Design review of the part built by this model. Coordinates are the model's own, in mm. A direction names the side the tool comes from. Coordinates: 2 decimals unless noted, no trailing zeros. Order: outer loops, then holes, each group sorted by start corner. A loop starts at its lowest first (then second) coordinate and runs counter-clockwise, first axis right, second up. Notation, with made-up numbers: M 88.5,71 L 113.5,71 A30 ccw 113.5,98 Z; hole C -17,52.25 d5. An arc over 180 degrees is marked long. Use CSV: the item, a comma, the result in double quotes.
Autodesk Fusion 360 part; units mm, degrees
sketch "Sketch1" plane through (0, 0, 0) normal (0, 1, 0) x (1, 0, 0)
  line L0 (0, 0) -> (6, 0)
  line L1 (6, 0) -> (6, -6)
  line L2 (6, -6) -> (0, -6)
  line L3 (0, -6) -> (0, 0)
  dimension "d1" = 6
  dimension "d2" = 6
extrude "Extrude1" add sketch "Sketch1" along normal blind 1.9
sketch "Sketch2" plane through (0, 1.9, 0) normal (0, 1, 0) x (-1, 0, 0)
  line L0 (0, 6) -> (-6, 6)
  line L1 (-6, 6) -> (-6, 0)
  line L2 (-6, 0) -> (0, 0)
  line L3 (0, 0) -> (0, 6)
  line L4 (-1.7485, 1.7053) -> (-4.3485, 1.7053)
  line L5 (-4.3485, 1.7053) -> (-4.3485, 4.3053)
  line L6 (-4.3485, 4.3053) -> (-1.7485, 4.3053)
  line L7 (-1.7485, 4.3053) -> (-1.7485, 1.7053)
  dimension "d5" = 2.6
  dimension "d6" = 2.6
extrude "Extrude2" add sketch "Sketch2" along normal blind 6.2 contours L4 L5 L6 L7
sketch "Sketch3" plane through (0, 0, 0) normal (0, -1, 0) x (1, 0, 0)
  line L0 (6, 6) -> (0, 6)
  line L1 (0, 6) -> (0, 0)
  line L2 (0, 0) -> (6, 0)
  line L3 (6, 0) -> (6, 6)
  line L4 (1.7485, 4.3053) -> (4.3485, 4.3053)
  line L5 (4.3485, 4.3053) -> (4.3485, 1.7053)
  line L6 (4.3485, 1.7053) -> (1.7485, 1.7053)
  line L7 (1.7485, 1.7053) -> (1.7485, 4.3053)
  point P0 (1.7485, 4.3053)
  point P1 (4.3485, 1.7053)
extrude "Extrude3" add sketch "Sketch3" along normal blind 1 contours L4 L5 L6 L7
(1) Add section C-C on y = 6.75. State the section outline as (x, z) points.
The answers:
outline,"M 1.75,1.71 L 4.35,1.71 L 4.35,4.31 L 1.75,4.31 Z"
(2) Clearance check with flat-ended pins moving along their axes: P1, Ø2, axis at x = 4, y = 3, coming from the +Z side; P2, Ø2, axis at y = 5.5, z = 2.5, coming from the -X side; P3, Ø2, axis at y = 3.5, z = 3, coming from the +X side; P4, Ø2, axis at y = 5.5, z = 0.5, coming from the +X side. State where each tip first meets the part, or that it passes through.
The answers:
P1,"stops at z = 4.31"
P2,"stops at x = 1.75"
P3,"stops at x = 4.35"
P4,"passes through"
(3) Wall thickness on probe 1 along Y at (x, z) = (5.65, 5.1); probe 2 along Z at (x, y) = (3.95, 6.25); probe 3 along X at (y, z) = (2, 1.9): over which ranges is each line inside the solid? List them lowest first.
The answers:
probe 1,"y = 0 to 1.9"
probe 2,"z = 1.71 to 4.31"
probe 3,"x = 1.75 to 4.35"
(4) Add section A-A on z = 3.95. State the section outline as (x, y) points.
The answers:
outline,"M 0,0 L 1.75,0 L 1.75,-1 L 4.35,-1 L 4.35,0 L 6,0 L 6,1.9 L 4.35,1.9 L 4.35,8.1 L 1.75,8.1 L 1.75,1.9 L 0,1.9 Z"
(5) Add section D-D on z = 4.8. State the section outline as (x, y) points.
The answers:
outline,"M 0,0 L 6,0 L 6,1.9 L 0,1.9 Z"
(6) Add section B-B on x = 3.8. State the section outline as (y, z) points, and give its area (3 significant figures).
The answers:
outline,"M -1,1.71 L 0,1.71 L 0,0 L 1.9,0 L 1.9,1.71 L 8.1,1.71 L 8.1,4.31 L 1.9,4.31 L 1.9,6 L 0,6 L 0,4.31 L -1,4.31 Z"
area,"30.1 mm2"
(7) For faces 1 (the face through (4.348, 5, 3)), 2 (the face through (3.1, -0.5, 1.705)), 3 (the face through (1.748, 5, 3)), 4 (the face through (4.348, -0.5, 3)), list the 3-axis set-ups (+Z, -Z, +X, -X, +Y, -Y) from which the entire face can be reached by the end or side of a thin tool; tool diameter is ignored.
The answers:
face 1,"+Z, -Z, +X, +Y"
face 2,"-Z, +X, -X, -Y"
face 3,"+Z, -Z, -X, +Y"
face 4,"+Z, -Z, +X, -Y"
